from build123d import *

# Parameters (mm, degrees)
EXTRUDE1_START = 84
SKETCH2_R      = 8.5
EXTRUDE1_DEPTH = 84
SKETCH3_R      = 7
EXTRUDE2_DEPTH = 23
EXTRUDE4_START = 6
EXTRUDE4_DEPTH = 10
EXTRUDE5_START = -6
EXTRUDE5_DEPTH = 10
CHAMFER1_SIZE  = 0.6135
CHAMFER2_SIZE  = 0.833333333
CHAMFER4_SIZE  = 0.75
CHAMFER5_SIZE  = 1.25
EXTRUDE6_DEPTH = 18.5
SKETCH7_R      = 2.5
EXTRUDE7_DEPTH = 7.62
SKETCH8_W      = 0.5
SKETCH8_H      = 0.7
CHAMFER6_SIZE  = 1.25


with BuildPart() as part:
    # Sketch1 → Revolve1 (revolve)
    with BuildSketch(Plane.XY, mode=Mode.PRIVATE) as revolve1_sk:
        Polygon((-6, 12.5), (-6, 0), (689, 0), (689, 8.5), (686.15, 8.5), (686.15, 8.15), (685, 8.15), (685, 8.5), (673, 8.5), (673, 12.5), (658.2, 12.5), (658.2, 12.25), (658, 12.25), (658, 12.5), (10, 12.5), (10, 12.25), (9.8, 12.25), (9.8, 12.5), align=None)
    revolve(revolve1_sk.sketch.rotate(Axis((-6, 0, 0), (1, 0, 0)), 270), axis=Axis((-6, 0, 0), (1, 0, 0)))

    # Sketch2 → Extrude1 (add)
    with BuildSketch(Plane.ZY.offset(6).offset(EXTRUDE1_START)):
        with Locations(Location((0, 0, 0), (0, 0, 180))):
            Circle(SKETCH2_R)
    extrude(amount=-EXTRUDE1_DEPTH)

    # Sketch3 → Extrude2 (add)
    with BuildSketch(Plane.ZY.offset(90)):
        Circle(SKETCH3_R)
    extrude(amount=EXTRUDE2_DEPTH)

    # Sketch5 → Extrude4 (cut)
    with BuildSketch(Plane(origin=(-6, 0, 0), x_dir=(0, 0, -1), z_dir=(1, 0, 0)).offset(EXTRUDE4_START)):
        with BuildLine():
            Line((9, 8.674675786), (9, -8.674675786))
            ThreePointArc((9, -8.674675786), (12.5, 0), (9, 8.674675786))
        make_face()
    extrude(amount=EXTRUDE4_DEPTH, mode=Mode.SUBTRACT)

    # Sketch6 → Extrude5 (cut)
    with BuildSketch(Plane(origin=(-6, 0, 0), x_dir=(0, -1, 0), z_dir=(-1, 0, 0)).offset(EXTRUDE5_START)):
        with BuildLine():
            Line((-8.674675786, 9), (8.674675786, 9))
            ThreePointArc((8.674675786, 9), (0, 12.5), (-8.674675786, 9))
        make_face()
    extrude(amount=-EXTRUDE5_DEPTH, mode=Mode.SUBTRACT)

    # Chamfer1
    chamfer1_edges = [part.edges().sort_by_distance(p)[0] for p in [
        (-90, 0, 8.5),
    ]]
    chamfer(chamfer1_edges, length=CHAMFER1_SIZE)

    # Chamfer2
    chamfer2_edges = [part.edges().sort_by_distance(p)[0] for p in [
        (-113, 0, -7),
    ]]
    chamfer(chamfer2_edges, length=CHAMFER2_SIZE)

    # Chamfer4
    chamfer4_edges = [part.edges().sort_by_distance(p)[0] for p in [
        (689, 0, 8.5),
    ]]
    chamfer(chamfer4_edges, length=CHAMFER4_SIZE)

    # Chamfer5
    chamfer5_edges = [part.edges().sort_by_distance(p)[0] for p in [
        (673, 0, 12.5),
    ]]
    chamfer(chamfer5_edges, length=CHAMFER5_SIZE)

    # Sketch4 → Extrude6 (cut)
    with BuildSketch(Plane.ZY.offset(113)):
        with BuildLine():
            Line((7.071067812, 2.5), (4.5, 2.5))
            Line((4.5, 2.5), (4.5, -2.5))
            Line((4.5, -2.5), (7.071067812, -2.5))
            ThreePointArc((7.071067812, -2.5), (7.5, 0), (7.071067812, 2.5))
        make_face()
    extrude(amount=-EXTRUDE6_DEPTH, mode=Mode.SUBTRACT)

    # Sketch7 → Extrude7 (cut)
    with BuildSketch(Plane.XY.offset(4.5)):
        with Locations((-94.5, 0)):
            Circle(SKETCH7_R)
    extrude(amount=EXTRUDE7_DEPTH, mode=Mode.SUBTRACT)

    # Sketch8 → Cut-Revolve1 (revolve, cut)
    with BuildSketch(Plane(origin=(0, 0, 0), x_dir=(1, 0, 0), z_dir=(0, 1, 0))):
        with Locations((-70.75, 8.15)):
            Rectangle(SKETCH8_W, SKETCH8_H)
    revolve(axis=Axis((0, 0, 0), (-1, 0, 0)), mode=Mode.SUBTRACT)

    # Chamfer6
    chamfer6_edges = [part.edges().sort_by_distance(p)[0] for p in [
        (-6, 0, 12.5),
    ]]
    chamfer(chamfer6_edges, length=CHAMFER6_SIZE)


solid = part.part
Geometry check sheet. Reference: the model listing, model coordinates, mm. A direction names the side the tool comes from. Give positions to 0.01 mm unless a question says otherwise; leave off trailing zeros. Write each loop counter-clockwise with the first axis right and the second up, starting at its lowest first coordinate (ties: lowest second). Pieces come first, ordered by that corner, then holes.
1) Cross-section at A-A (x = 527). Record the boundary of the cut face in (y, z).
Values follow:
outline: circle Ø25 at (0, 0)
2) Go/stop test with flat-tipped pins: pin 1 Ø8 at (x, y) = (5.5, 2) entering from -Z; pin 2 Ø6 at (y, z) = (8, 9.5) entering from +X; pin 3 Ø2 at (y, z) = (9.5, 7) entering from -X. Record where each tip stops, or that it passes through.
Values follow:
pin 1: stops at z = -9
pin 2: stops at x = 673
pin 3: stops at x = -6
3) Release check for a two-part mould opening along X. For faces 5 (the face through (689, 0, 0)), 6 (the face through (-70.5, 7, 4)), 7 (the face through (329.464, 3.755, -11.923)) record: released by +X, released by -X, zero draft, split by the parting line, or undercut.
Values follow:
face 5: released by +X
face 6: undercut
face 7: zero draft
4) Thickness scan on line 1 (X direction, y = -3.75, z = 10.25); line 2 (Z direction, x = 539.5, y = -2.75); line 3 (Z direction, x = 527, y = -5.25). Record the ranges inside material, lowest first.
Values follow:
line 1: x = -6 to 0, 10 to 673
line 2: z = -12.19 to 12.19
line 3: z = -11.34 to 11.34
5) Set-up check for faces 1 (the face through (-6, 8, -4)), 2 (the face through (-70.746, -7.734, 1.015)), 3 (the face through (664.88, 3.755, -11.923)), 4 (the face through (687.185, 8.428, 1.107)): record each of +Z, -Z, +X, -X, +Y, -Y from which the full face is reachable in a straight line by a thin tool's end or side.
Values follow:
face 1: -X
face 2: none
face 3: +X, -X
face 4: +X
